Print and shaded views of the part. All mm, measured from the part's lowest x, y and z. Round coordinates to 2 decimals unless told otherwise and drop trailing zeros. Loops run counter-clockwise (first coordinate to the right, second up) from the corner with the lowest first, then second, coordinate; pieces in that order, holes last. Notation, with made-up numbers: (87.25, 27) - (145.25, 27) arc R22 ccw to (145.25, 35) - close; hole circle Ø4 at (-5.75, 51.5). An arc over 180 degrees is marked (long way). Use one line per item in the form item = value. Start each with the question number.
Q1. Pin check, flat tips, straight feed: pin 1 (1.5 mm diameter, centred on x = 13, z = 2, fed in from -Y); pin 2 (1.5 mm diameter, centred on y = 25, z = 1.5, fed in from +X); pin 3 (1.5 mm diameter, centred on y = 22.5, z = 2, fed in from -X); pin 4 (1.5 mm diameter, centred on x = 54.5, z = 2, fed in from -Y). Stop position of each tip, or through.
Q2. Drill centre lines: line 1 (Y direction, x = 40, z = 1.1); line 2 (X direction, y = 35.5, z = 1.05); line 3 (Y direction, x = 51, z = 2). Where is each one in solid material? Low to high.
Q3. Saw through at D-D (y = 50). Give the cut face in (x, z).
Q4. Saw through at B-B (x = 30). Give the cut face in (y, z).
Q5. Saw through at A-A (y = 10). Give the cut face in (x, z).
Q6. Saw through at C-C (z = 1.6). Give the cut face in (x, y).
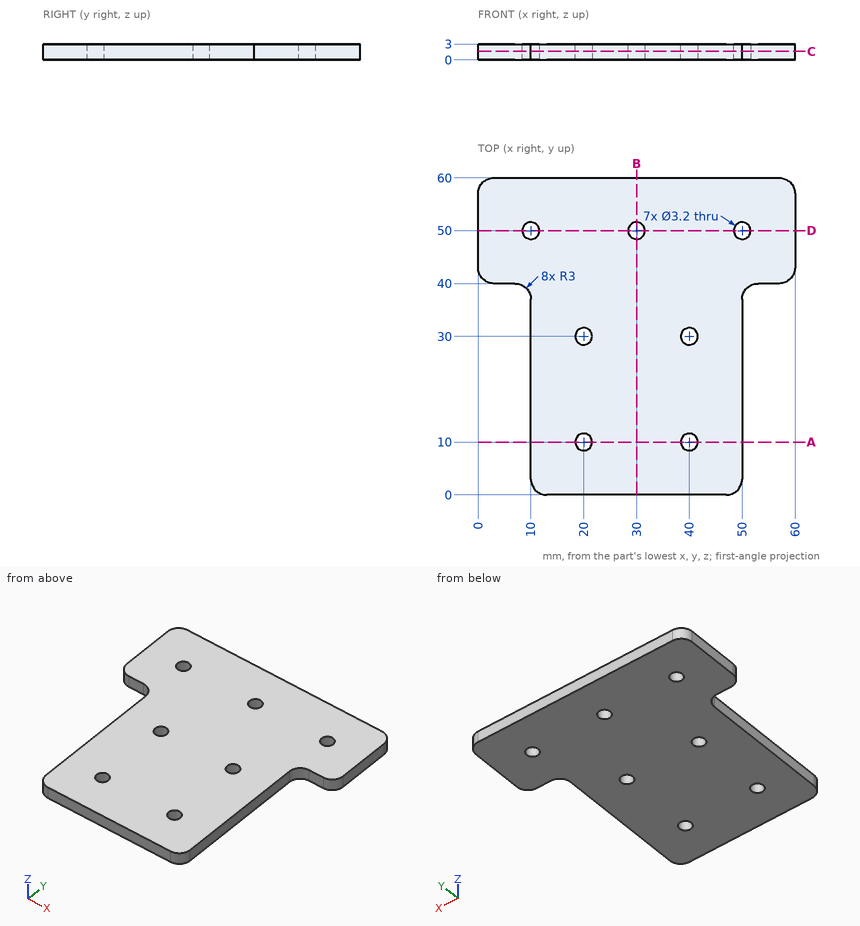
Report:
q1.pin_1 = 0
q1.pin_2 = 50
q1.pin_3 = 10
q1.pin_4 = 40
q2.line_1 = 0 to 8.4, 11.6 to 28.4, 31.6 to 60
q2.line_2 = 10 to 50
q2.line_3 = 39.24 to 48.75, 51.25 to 60
q3.outline = (0, 0) - (8.4, 0) - (8.4, 3) - (0, 3) - close; (11.6, 0) - (28.4, 0) - (28.4, 3) - (11.6, 3) - close; (31.6, 0) - (48.4, 0) - (48.4, 3) - (31.6, 3) - close; (51.6, 0) - (60, 0) - (60, 3) - (51.6, 3) - close
q4.outline = (0, 0) - (48.4, 0) - (48.4, 3) - (0, 3) - close; (51.6, 0) - (60, 0) - (60, 3) - (51.6, 3) - close
q5.outline = (10, 0) - (18.4, 0) - (18.4, 3) - (10, 3) - close; (21.6, 0) - (38.4, 0) - (38.4, 3) - (21.6, 3) - close; (41.6, 0) - (50, 0) - (50, 3) - (41.6, 3) - close
q6.outline = (0, 43) arc R3 ccw to (3, 40) - (7, 40) arc R3 cw to (10, 37) - (10, 3) arc R3 ccw to (13, 0) - (47, 0) arc R3 ccw to (50, 3) - (50, 37) arc R3 cw to (53, 40) - (57, 40) arc R3 ccw to (60, 43) - (60, 57) arc R3 ccw to (57, 60) - (3, 60) arc R3 ccw to (0, 57) - close; hole circle Ø3.2 at (10, 50); hole circle Ø3.2 at (20, 10); hole circle Ø3.2 at (20, 30); hole circle Ø3.2 at (30, 50); hole circle Ø3.2 at (40, 10); hole circle Ø3.2 at (40, 30); hole circle Ø3.2 at (50, 50)
